Could you check a few things on this model? Use its own coordinates, in mm. Coordinates: 2 decimals unless noted, no trailing zeros. Order: outer loops, then holes, each group sorted by start corner. A loop starts at its lowest first (then second) coordinate and runs counter-clockwise, first axis right, second up. Notation, with made-up numbers: M -30.75,-22.75 L 9.25,-22.75 A27 cw 9.25,15.25 Z; hole C 43,0.25 d1. An arc over 180 degrees is marked long. Put each result on its own line as item: value. Start each with the question number.
```python
from build123d import *

# Parameters (mm, degrees)
SKETCH_R   = 4.05
SKETCH_R_2 = 2.6
SKETCH_R_3 = 3.2
SKETCH_R_4 = 2.4
PAD_DEPTH  = 3
FILLET_R   = 8


with BuildPart() as part:
    # Sketch → Pad (new body)
    with BuildSketch(Plane.XY):
        Polygon((-182.5, 100), (-182.5, 0), (182.5, 0), (182.5, 25), (102.5, 25), (102.5, 100), align=None)
        with Locations((-14.5, 87.7)):
            Circle(SKETCH_R, mode=Mode.SUBTRACT)
        with Locations((-64.5, 67.7)):
            Circle(SKETCH_R, mode=Mode.SUBTRACT)
        with Locations((35.5, 67.7)):
            Circle(SKETCH_R, mode=Mode.SUBTRACT)
        with Locations((-32.75, 87.7)):
            Circle(SKETCH_R_2, mode=Mode.SUBTRACT)
        with Locations((3.75, 87.7)):
            Circle(SKETCH_R_2, mode=Mode.SUBTRACT)
        with Locations((19.25, 67.7)):
            Circle(SKETCH_R_3, mode=Mode.SUBTRACT)
        with Locations((51.75, 67.7)):
            Circle(SKETCH_R_3, mode=Mode.SUBTRACT)
        with Locations((-80.75, 67.7)):
            Circle(SKETCH_R_3, mode=Mode.SUBTRACT)
        with Locations((-48.25, 67.7)):
            Circle(SKETCH_R_3, mode=Mode.SUBTRACT)
        with Locations((-169.5, 13)):
            Circle(SKETCH_R_4, mode=Mode.SUBTRACT)
        with Locations((169.5, 13)):
            Circle(SKETCH_R_4, mode=Mode.SUBTRACT)
        with Locations((20, 13)):
            Circle(SKETCH_R_4, mode=Mode.SUBTRACT)
        with Locations((-20, 13)):
            Circle(SKETCH_R_4, mode=Mode.SUBTRACT)
    extrude(amount=PAD_DEPTH)

    # Fillet
    fillet_edges = [part.edges().sort_by_distance(p)[0] for p in [
        (102.5, 100, 1.5),
        (102.5, 25, 1.5),
        (182.5, 25, 1.5),
    ]]
    fillet(fillet_edges, radius=FILLET_R)


solid = part.part
```
Item 1: If we section it at A-A on y = 67.7: Write out the boundary of the cut face in (x, z), then the cut area to 3 significant figures.
Item 2: I need wall thicknesses on probe 1 along Y at (x, z) = (35.5, 1.85); probe 2 along Y at (x, z) = (-80.75, 1.9); probe 3 along X at (y, z) = (86.5, 0.6). Which ranges of each line are inside material? Lowest first, please.
Item 3: If we section it at D-D on x = -14.5: Write out the boundary of the cut face in (y, z), then the cut area to 3 significant figures.
Item 4: If we mould it in two halves opening along Y, with no side actions, what happens to faces 1 (the flat face through (-43, 51, 0)), 2 (the cylindrical face through (37.369, 64.107, 1.479)), 3 (the cylindrical face through (100.094, 97.719, 1.521))? For each: released by +Y, released by -Y, zero draft, split by the parting line, or undercut.
Item 5: If we section it at B-B on x = 51.75: Write out the boundary of the cut face in (y, z).
Item 6: If we section it at C-C on z = 1: State how many separate pieces and enclosed holes the cut face has, then the cut area to 3 significant figures.
Item 7: For pin 1 Ø0.9 at (y, z) = (62.5, 2) entering from +X, with a flat end and sliding along its axis, tell me the tip position at first contact or that it passes through.
Geometry check:
1. outline: M -182.5,0 L -83.95,0 L -83.95,3 L -182.5,3 Z; M -77.55,0 L -68.55,0 L -68.55,3 L -77.55,3 Z; M -60.45,0 L -51.45,0 L -51.45,3 L -60.45,3 Z; M -45.05,0 L 16.05,0 L 16.05,3 L -45.05,3 Z; M 22.45,0 L 31.45,0 L 31.45,3 L 22.45,3 Z; M 39.55,0 L 48.55,0 L 48.55,3 L 39.55,3 Z; M 54.95,0 L 102.5,0 L 102.5,3 L 54.95,3 Z
1. area: 730 mm²
2. probe 1: y = 0 to 63.65, 71.75 to 100
2. probe 2: y = 0 to 64.5, 70.9 to 100
2. probe 3: x = -182.5 to -35.06, -30.44 to -18.37, -10.63 to 1.44, 6.06 to 102.5
3. outline: M 0,0 L 83.65,0 L 83.65,3 L 0,3 Z; M 91.75,0 L 100,0 L 100,3 L 91.75,3 Z
3. area: 276 mm²
4. face 1: zero draft
4. face 2: undercut
4. face 3: released by +Y
5. outline: M 0,0 L 64.5,0 L 64.5,3 L 0,3 Z; M 70.9,0 L 100,0 L 100,3 L 70.9,3 Z
6. separate pieces: 1
6. enclosed holes: 13
6. area: 30,100 mm²
7. pin 1: stops at x = 102.5
